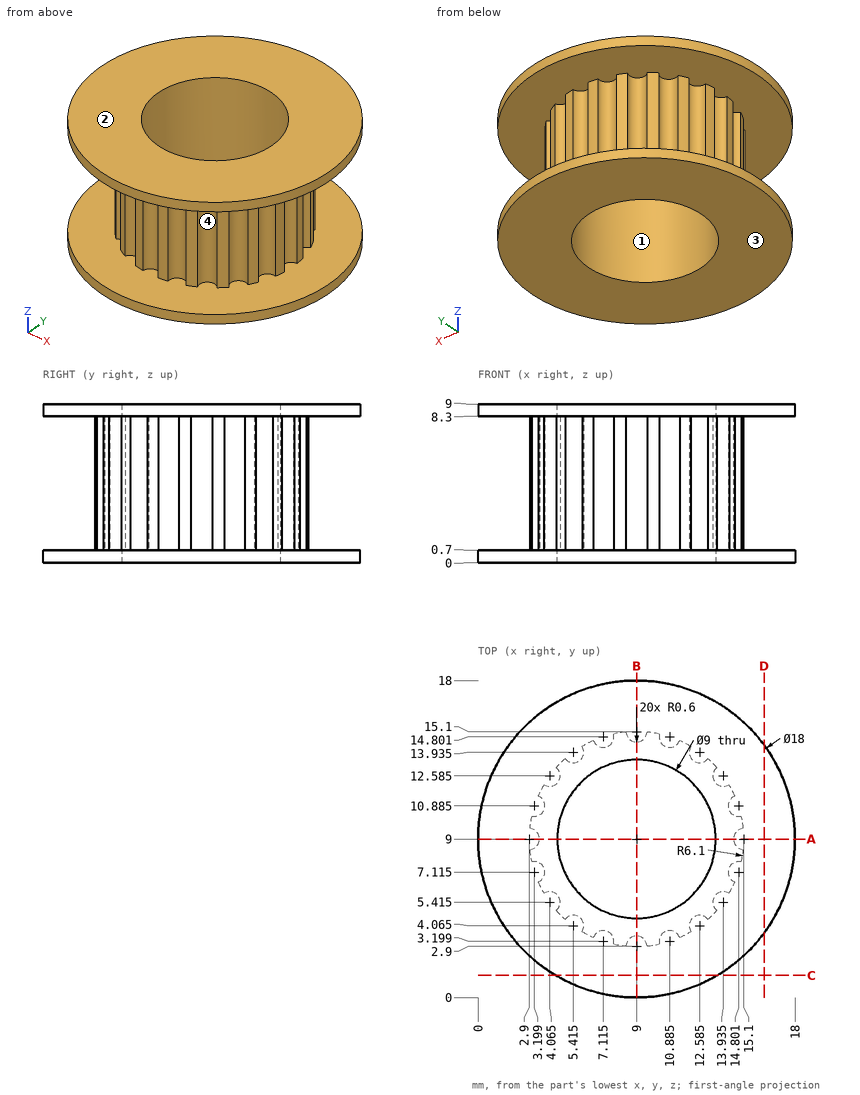
Study the drawing (mm; zero at the part's minimum x, y, z) and answer. A direction names the side the tool comes from. Give positions to 0.01 mm unless a question says otherwise; leave off trailing zeros. Loops run counter-clockwise (first coordinate to the right, second up) from the corner with the lowest first, then second, coordinate; pieces in that order, holes last. Notation, with made-up numbers: (-30, 74) - (-3, 74) arc R35 ccw to (-3, 108) - close; hole circle Ø1 at (-8.5, 2.25). An arc over 180 degrees is marked (long way). Return JSON: item names as keys, results as strings. Group by question number.
1. Find section D-D (x = 16.25). Write down the section's boundary in (y, z).
2. Which of the six approach directions +Z, -Z, +X, -X, +Y, -Y give full straight-line access (tool end or side, diameter ignored) to the marked faces 3 and 4?
3. Given pin 1 Ø3 at (x, z) = (13.5, 1) entering from -Y (1 decimal); pin 2 Ø1.5 at (y, z) = (8.5, 2.5) entering from +X; pin 3 Ø1.5 at (x, y) = (12.5, 7.5) entering from -Z, each flat-ended and moving along its own axis, determine where each tip first touches the part or whether it passes through.
4. Straight lines are drawn through the part: line 1 (Z direction, x = 5.75, y = 13.5); line 2 (Y direction, x = 8, z = 7); line 3 (Y direction, x = 8.5, z = 7.5) (1 decimal). For each, find the intervals that lie inside material, in ascending order. Write a range as [from, to].
5. Determine the mould class of the marked faces 1 and 2 for opening direction Y: pulls with the +Y half, pulls with the -Y half, needs draft (parallel to the pull), parting line crosses it, or undercut.
6. Find section A-A (y = 9). Write down the section's boundary in (x, z).
7. Find section C-C (y = 1.25). Write down the section's boundary in (x, z) (1 decimal).
Verdict:
{
 "1": {"outline": "(3.67, 0) - (14.33, 0) - (14.33, 0.7) - (3.67, 0.7) - close; (3.67, 8.3) - (14.33, 8.3) - (14.33, 9) - (3.67, 9) - close"},
 "2": {"face 3": "-Z, +X, -X, +Y, -Y", "face 4": "none"},
 "3": {"pin 1": "stops at y = 0.5", "pin 2": "stops at x = 15.07", "pin 3": "stops at z = 0"},
 "4": {"line 1": "z = [0, 0.7], [8.3, 9]", "line 2": "y = [2.98, 4.61], [13.39, 15.02]", "line 3": "y = [3.2, 4.5], [13.5, 14.8]"},
 "5": {"face 1": "undercut", "face 2": "needs draft"},
 "6": {"outline": "(0, 0) - (4.5, 0) - (4.5, 9) - (0, 9) - (0, 8.3) - (3.5, 8.3) - (3.5, 0.7) - (0, 0.7) - close; (13.5, 0) - (18, 0) - (18, 0.7) - (14.5, 0.7) - (14.5, 8.3) - (18, 8.3) - (18, 9) - (13.5, 9) - close"},
 "7": {"outline": "(4.4, 0) - (13.6, 0) - (13.6, 0.7) - (4.4, 0.7) - close; (4.4, 8.3) - (13.6, 8.3) - (13.6, 9) - (4.4, 9) - close"}
}
